Verification items for the finished model (mm, model axes). A direction names the side the tool comes from. Give positions to 0.01 mm unless a question says otherwise; leave off trailing zeros. Order: outer loops, then holes, each group sorted by start corner. A loop starts at its lowest first (then second) coordinate and runs counter-clockwise, first axis right, second up.
(1) Sectioned sample at B-B on y = 7. Record the cut outline in (x, z), plus the area to 3 significant figures.
(2) Gauge pin test, flat ends, axial feed: pin 1 (3.5 mm diameter, centred on y = 6, z = 7.5, fed in from +X); pin 2 (6 mm diameter, centred on x = 19, y = 7.5, fed in from +Z); pin 3 (0.9 mm diameter, centred on x = 34.5, z = 10, fed in from +Y). Record the tip position at first contact, or that the pin passes through.
(3) Mould release check, pull along Z, two halves, no side actions. Record for faces 5 (the face through (25.2, 1.6, 5)), 6 (the face through (33, 0, 12)), 7 (the face through (1, -6, -6)), 8 (the face through (33.955, -4.145, 4.029)): pulls with the +Z half, pulls with the -Z half, needs draft (parallel to the pull), parting line crosses it, or undercut.
(4) Scan lines: L1, parallel to Y at x = 21.5, z = 0; L2, parallel to X at y = 4.75, z = -8.25; L3, parallel to Y at x = 14, z = 2.75. Record each from-to range of solid material in increasing order.
(5) Sectioned sample at A-A on x = 42.5. Record the cut outline in (y, z), plus the area to 3 significant figures.
(6) Sectioned sample at C-C on z = 8. Record the cut outline in (x, y).
(7) Access from +Z, -Z, +X, -X, +Y, -Y to the whole of each face (thin tool, end or side, straight path). Record for faces 1 (the face through (34, 10, -1)), 2 (the face through (1, -6, 7)), 3 (the face through (1, 7, 7)), 4 (the face through (34, -1, -10)).
```python
from build123d import *

# Parameters (mm, degrees)
CROQUIS1_R              = 12
SALIENTE_EXTRUIR1_DEPTH = 66
CROQUIS2_R              = 5.25
CORTAR_EXTRUIR1_DEPTH   = 50
CORTAR_EXTRUIR3_DEPTH   = 65
REDONDEO1_R             = 1


with BuildPart() as part:
    # Croquis1 → Saliente-Extruir1 (new body)
    with BuildSketch(Plane(origin=(0, 0, 0), x_dir=(0, 0, -1), z_dir=(1, 0, 0))):
        Circle(CROQUIS1_R)
    extrude(amount=SALIENTE_EXTRUIR1_DEPTH)

    # Croquis2 → Cortar-Extruir1 (cut)
    with BuildSketch(Plane.ZY):
        Circle(CROQUIS2_R)
    extrude(amount=-CORTAR_EXTRUIR1_DEPTH, mode=Mode.SUBTRACT)

    # Croquis3 → Cortar-Extruir3 (cut)
    with BuildSketch(Plane(origin=(66, 0, 0), x_dir=(0, 0, -1), z_dir=(1, 0, 0))):
        with BuildLine():
            ThreePointArc((-1, 11.958260743), (-8.485281374, 8.485281374), (-11.958260743, 1))
            Line((-11.958260743, 1), (-9, 1))
            ThreePointArc((-9, 1), (-4.056739766, 4.056739766), (-1, 9))
            Line((-1, 9), (-1, 11.958260743))
        make_face()
        with BuildLine():
            Line((9, 1), (11.958260743, 1))
            ThreePointArc((11.958260743, 1), (8.485281374, 8.485281374), (1, 11.958260743))
            Line((1, 11.958260743), (1, 9))
            ThreePointArc((1, 9), (4.049951004, 4.049951004), (9, 1))
        make_face()
        with BuildLine():
            ThreePointArc((9, -1), (4.106809031, -4.106809031), (1, -9))
            Line((1, -9), (1, -11.958260743))
            ThreePointArc((1, -11.958260743), (8.485281374, -8.485281374), (11.958260743, -1))
            Line((11.958260743, -1), (9, -1))
        make_face()
        with BuildLine():
            ThreePointArc((-11.958260743, -1), (-8.485281374, -8.485281374), (-1, -11.958260743))
            Line((-1, -11.958260743), (-1, -9))
            ThreePointArc((-1, -9), (-4.086933884, -4.086933884), (-9, -1))
            Line((-9, -1), (-11.958260743, -1))
        make_face()
    extrude(amount=-CORTAR_EXTRUIR3_DEPTH, mode=Mode.SUBTRACT)

    # Redondeo1
    redondeo1_edges = [part.edges().sort_by_distance(p)[0] for p in [
        (0, 0, -5.25),
    ]]
    fillet(redondeo1_edges, radius=REDONDEO1_R)

    # Croquis8 → Cortar-Revolución1 (revolve, cut)
    with BuildSketch(Plane.XY):
        with BuildLine():
            Line((50, 0), (62.972700569, 0))
            ThreePointArc((62.972700569, 0), (56.963621034, 3.875725549), (50, 5.5))
            Line((50, 5.5), (50, 0))
        make_face()
    revolve(axis=Axis((50, 0, 0), (1, 0, 0)), mode=Mode.SUBTRACT)


solid = part.part
```
Ans:
1. outline: (0, -9.75) - (1, -9.75) - (1, -1.86) - (66, -1.86) - (66, 1.87) - (1, 1.87) - (1, 9.75) - (0, 9.75) - close
1. area: 262 mm2
2. pin 1: stops at x = 1
2. pin 2: stops at z = 3.63
2. pin 3: stops at y = 1
3. face 5: undercut
3. face 6: parting line crosses it
3. face 7: needs draft
3. face 8: pulls with the +Z half
4. L1: y = -12 to -5.25, 5.25 to 12
4. L2: x = 0 to 1
4. L3: y = -5.65 to -4.47, 4.47 to 5.59
5. outline: (-11.96, -1) - (-9, -1) arc R13.3 cw to (-1, -9) - (-1, -11.96) arc R12 ccw to (1, -11.96) - (1, -9) arc R12.58 cw to (9, -1) - (11.96, -1) arc R12 ccw to (11.96, 1) - (9, 1) arc R12.66 cw to (1, 9) - (1, 11.96) arc R12 ccw to (-1, 11.96) - (-1, 9) arc R13.04 cw to (-9, 1) - (-11.96, 1) arc R12 ccw to start; hole circle Ø10.5 at (0, 0)
5. area: 93.4 mm2
6. outline: (0, -8.94) - (1, -8.94) - (1, -1.4) - (66, -1.4) - (66, 1.38) - (1, 1.38) - (1, 8.94) - (0, 8.94) - close
7. face 1: -Z, +X, +Y
7. face 2: +Z, +X, -Y
7. face 3: +Z, +X, +Y
7. face 4: -Z, +X, -Y
